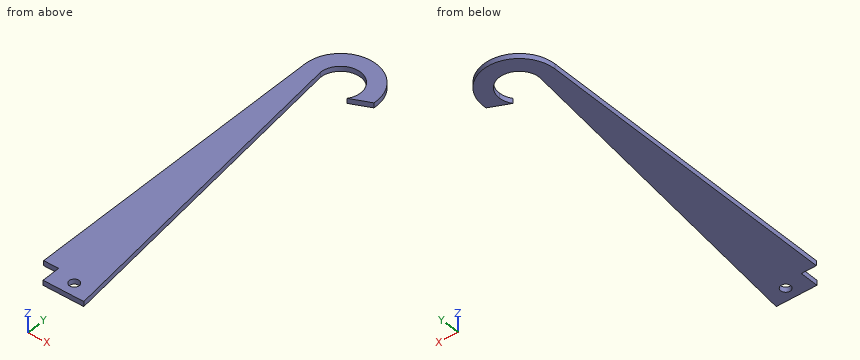
from build123d import *

# Parameters (mm, degrees)
SKETCH1_R           = 6.35
BOSS_EXTRUDE1_DEPTH = 6.35


with BuildPart() as part:
    # Sketch1 → Boss-Extrude1 (new body)
    with BuildSketch(Plane.XY):
        with BuildLine():
            Line((3.331127109, 389.92455355), (27.90992579, 401.162728042))
            ThreePointArc((27.90992579, 401.162728042), (-15.607198263, 450.028916488), (-62.759573024, 404.660447113))
            Line((-62.759573024, 404.660447113), (-62.759573024, 6.090179643))
            Line((-62.759573024, 6.090179643), (-43.715258354, 6.090179643))
            Line((-43.715258354, 6.090179643), (-43.715258354, -17.785820357))
            Line((-43.715258354, -17.785820357), (8.125653236, -17.785820357))
            Line((8.125653236, -17.785820357), (-42.757358599, 404.660447113))
            ThreePointArc((-42.757358599, 404.660447113), (-17.357358599, 430.060447113), (8.042641401, 404.660447113))
            ThreePointArc((8.042641401, 404.660447113), (6.83610681, 396.925058855), (3.331127109, 389.92455355))
        make_face()
        with Locations((-17.357358599, -1.739552887)):
            Circle(SKETCH1_R, mode=Mode.SUBTRACT)
    extrude(amount=BOSS_EXTRUDE1_DEPTH)


solid = part.part
Work out the finished part from the listing and answer in its coordinate system (mm). Round coordinates to 2 decimals unless told otherwise and drop trailing zeros. Loops run counter-clockwise (first coordinate to the right, second up) from the corner with the lowest first, then second, coordinate; pieces in that order, holes last. Notation, with made-up numbers: (60, -13.75) - (103, -13.75) arc R31 cw to (103, 20.25) - close; hole circle Ø10 at (-5, 35.5). An arc over 180 degrees is marked (long way). One line per item, written item: value.
Q1. Each of these flat-tipped pins is pushed along its axis until it touches: pin 1 Ø3 at (x, z) = (-57, 2.5) entering from -Y; pin 2 Ø11.5 at (x, y) = (-17.36, -1.74) entering from +Z; pin 3 Ø3 at (y, z) = (309, 0.5) entering from +X; pin 4 Ø1 at (y, z) = (322.5, 4.5) entering from +X. Where does it stop, or does it pass through?
Check values:
pin 1: y = 6.09
pin 2: through
pin 3: x = -31.05
pin 4: x = -32.8
Q2. Find section D-D on y = 138. Give the vertices of the cut face in (x, z), and give its area (3 significant figures).
Check values:
outline: (-62.76, 0) - (-10.64, 0) - (-10.64, 6.35) - (-62.76, 6.35) - close
area: 331 mm2
Q3. Find section B-B on x = -35. Give the vertices of the cut face in (y, z), and give its area (3 significant figures).
Check values:
outline: (-17.79, 0) - (340.26, 0) - (340.26, 6.35) - (-17.79, 6.35) - close; (422.93, 0) - (446.49, 0) - (446.49, 6.35) - (422.93, 6.35) - close
area: 2,420 mm2
Q4. Find section A-A on x = -16.5. Give the vertices of the cut face in (y, z).
Check values:
outline: (-17.79, 0) - (-8.03, 0) - (-8.03, 6.35) - (-17.79, 6.35) - close; (4.55, 0) - (186.66, 0) - (186.66, 6.35) - (4.55, 6.35) - close; (430.05, 0) - (450.05, 0) - (450.05, 6.35) - (430.05, 6.35) - close
Q5. Find section C-C on z = 4.25. Give the vertices of the cut face in (x, y).
Check values:
outline: (-62.76, 6.09) - (-43.72, 6.09) - (-43.72, -17.79) - (8.13, -17.79) - (-42.76, 404.66) arc R25.4 cw (long way) to (3.33, 389.92) - (27.91, 401.16) arc R45.4 ccw (long way) to (-62.76, 404.66) - close; hole circle Ø12.7 at (-17.36, -1.74)
Q6. Straight lines are drawn through the part: probe 1 along X at (y, z) = (11.5, 5); probe 2 along X at (y, z) = (426.5, 1.25); probe 3 along Y at (x, z) = (15.5, 5). For each, find the intervals that lie inside material, in ascending order.
Check values:
probe 1: -62.76 to 4.6
probe 2: -57.16 to -30.33, -4.39 to 22.45
probe 3: 395.49 to 435.99
